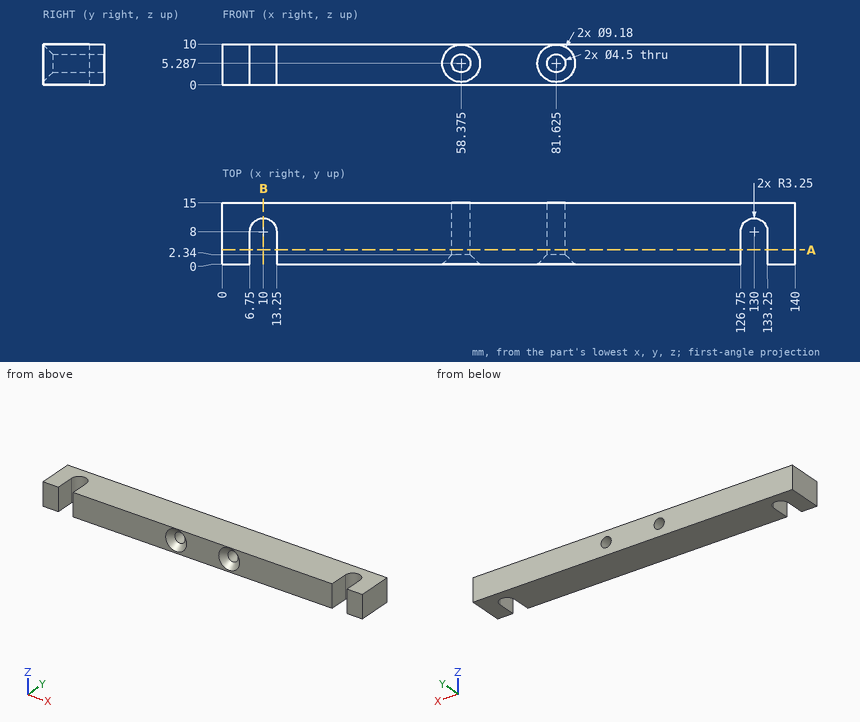
Can you work these out from the drawing? Everything is in mm from the part's minimum corner. Coordinates: 2 decimals unless noted, no trailing zeros. Order: outer loops, then holes, each group sorted by start corner. A loop starts at its lowest first (then second) coordinate and runs counter-clockwise, first axis right, second up. Notation, with made-up numbers: M -31,6 L 18,6 A31 ccw 18,33 Z; hole C 26.5,60 d5. An arc over 180 degrees is marked long. Answer as CSV lines item,"result". Start each with the question number.
1. I want a section at B-B, the plane x = 10. Write out the boundary of the cut face in (y, z).
2. I want a section at A-A, the plane y = 3.5. Count the separate pieces of the cut face and the enclosed holes in it, and give its area (3 significant figures).
3. For pin 1 (1.5 mm diameter, centred on x = 39.5, z = 6, fed in from -Y), with a flat end and sliding along its axis, tell me the tip position at first contact or that it passes through.
4. I need wall thicknesses on line 1 (X direction, y = 5, z = 9.25); line 2 (X direction, y = 10.5, z = 6.75) (1 decimal); line 3 (X direction, y = 11.5, z = 4.25). Which ranges of each line are inside material? Lowest first, please. Write a range as [from, to].
Recorded:
1,outline,"M 11.25,0 L 15,0 L 15,10 L 11.25,10 Z"
2,separate pieces,"3"
2,enclosed holes,"2"
2,area,"1,240 mm2"
3,pin 1,"stops at y = 0"
4,line 1,"x = [0, 6.75], [13.25, 126.75], [133.25, 140]"
4,line 2,"x = [0, 7.9], [12.1, 56.7], [60.1, 79.9], [83.3, 127.9], [132.1, 140]"
4,line 3,"x = [0, 56.38], [60.37, 79.63], [83.62, 140]"
